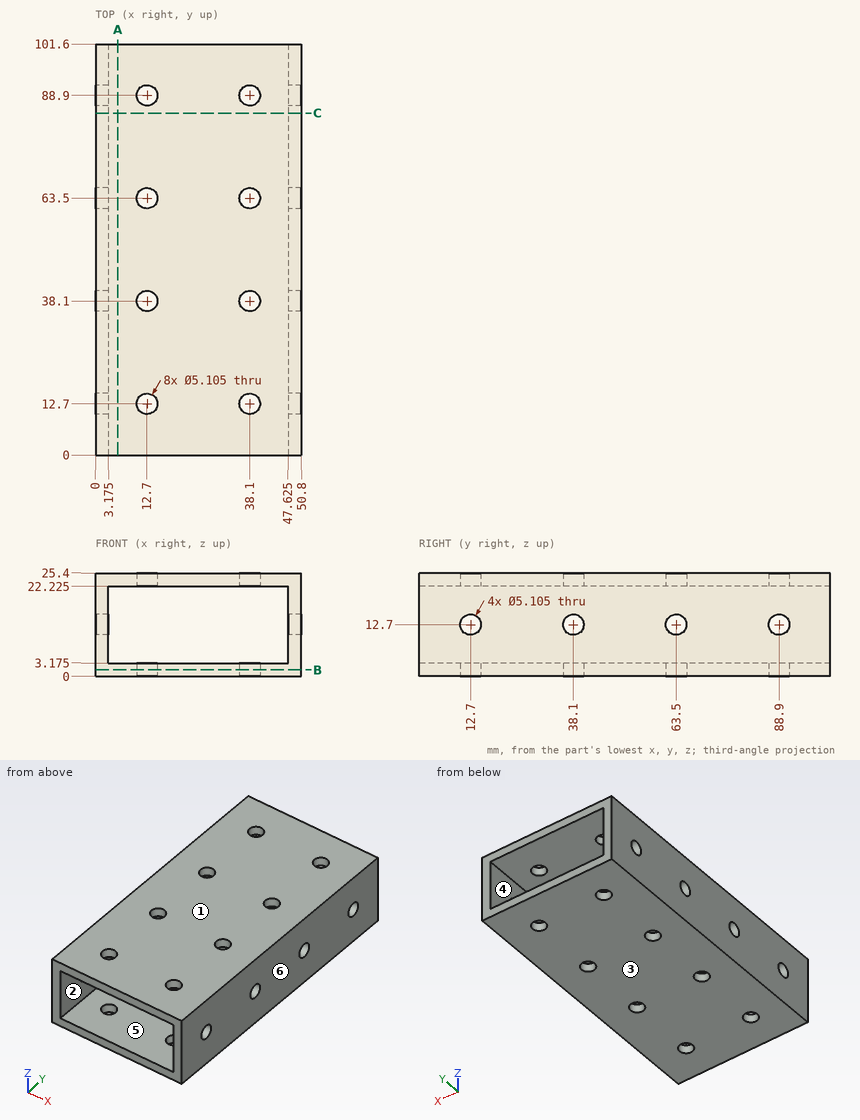
Could you check a few things on this drawing? It's one solid part, dimensions in mm from its lowest x, y, z. A direction names the side the tool comes from. Coordinates: 2 decimals unless noted, no trailing zeros. Order: outer loops, then holes, each group sorted by start corner. A loop starts at its lowest first (then second) coordinate and runs counter-clockwise, first axis right, second up. Notation, with made-up numbers: M 73.5,14 L 120.5,14 A17 cw 120.5,20 Z; hole C -19,23 d1. An arc over 180 degrees is marked long. Answer as a JSON object with one key per item and string values. Group by question number.
(1) I need wall thicknesses on probe 1 along X at (y, z) = (88.9, 24.15); probe 2 along Y at (x, z) = (38.1, 2); probe 3 along X at (y, z) = (71, 20.25) (1 decimal). Which ranges of each line are inside material? Lowest first, please.
(2) Suppose I cut it at C-C, the plane y = 84.5. Please give me the cut outline in (x, z) (1 decimal).
(3) Which directions (+Z, -Z, +X, -X, +Y, -Y) give clear straight access to the entire face, cutting with the end or side of a thin tool? Please do the marked faces 5 and 6.
(4) If we mould it in two halves opening along Z, with no side actions, what happens to the marked faces 1, 2, 3 and 4? For each: released by +Z, released by -Z, zero draft, split by the parting line, or undercut.
(5) Suppose I cut it at B-B, the plane z = 1.5. State how many separate pieces and enclosed holes the cut face has, then the cut area to 3 significant figures.
(6) Suppose I cut it at A-A, the plane x = 5.5. Please give me the cut outline in (y, z) (1 decimal), then the cut area to 3 significant figures.
Values found:
{
 "1": {"probe 1": "x = 0 to 10.15, 15.25 to 35.55, 40.65 to 50.8", "probe 2": "y = 0 to 10.15, 15.25 to 35.55, 40.65 to 60.95, 66.05 to 86.35, 91.45 to 101.6", "probe 3": "x = 0 to 3.2, 47.6 to 50.8"},
 "2": {"outline": "M 0,0 L 50.8,0 L 50.8,25.4 L 0,25.4 Z; hole M 3.2,3.2 L 47.6,3.2 L 47.6,22.2 L 3.2,22.2 Z"},
 "3": {"face 5": "+Y, -Y", "face 6": "+Z, -Z, +X, +Y, -Y"},
 "4": {"face 1": "released by +Z", "face 2": "undercut", "face 3": "released by -Z", "face 4": "undercut"},
 "5": {"separate pieces": "1", "enclosed holes": "8", "area": "5,000 mm^2"},
 "6": {"outline": "M 0,0 L 101.6,0 L 101.6,3.2 L 0,3.2 Z; M 0,22.2 L 101.6,22.2 L 101.6,25.4 L 0,25.4 Z", "area": "645 mm^2"}
}
